Source: CAD feature listing. Evaluate the final solid. Frame: model axes, mm. Face numbers are marked on the shaded views. Give positions to 0.01 mm unless a question says otherwise; leave off trailing zeros. Loops run counter-clockwise (first coordinate to the right, second up) from the corner with the lowest first, then second, coordinate; pieces in that order, holes last.
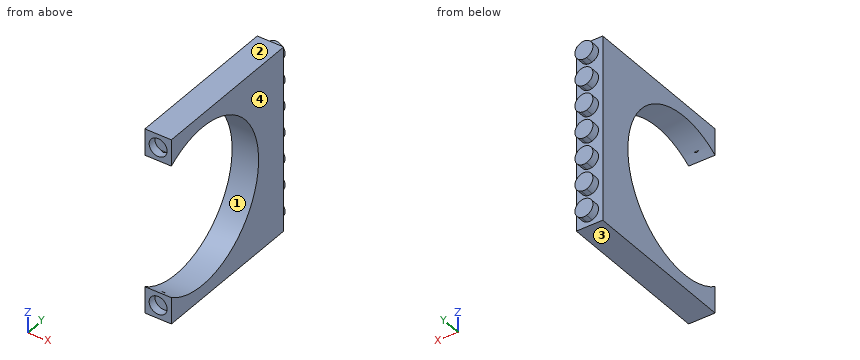
Autodesk Inventor part; units mm, degrees
ref_plane "YZ Plane" through (0, 0, 0) normal (1, 0, 0) x (0, 1, 0)
ref_plane "XZ Plane" through (0, 0, 0) normal (0, 1, 0) x (-1, 0, 0)
ref_plane "XY Plane" through (0, 0, 0) normal (0, 0, 1) x (1, 0, 0)
sketch "草圖1" plane through (0, 0, 0) normal (0, 1, 0) x (-1, 0, 0)
  line L0 (5, 0) -> (0, 0)
  line L1 (0, 0) -> (0, -35)
  line L2 (0, -35) -> (5, -35)
  line L3 (5, -35) -> (5, 0)
  circle A0 centre (2.5, -2.5) radius 1.7
  circle A1 centre (2.5, -7.5) radius 1.7
  circle A2 centre (2.5, -12.5) radius 1.7
  circle A3 centre (2.5, -17.5) radius 1.7
  circle A4 centre (2.5, -22.5) radius 1.7
  circle A5 centre (2.5, -27.5) radius 1.7
  circle A6 centre (2.5, -32.5) radius 1.7
  line L4 (5, -5) -> (0, -5)
  line L5 (5, -30) -> (0, -30)
  dimension "d0" = 5
  dimension "d1" = 35
  dimension "d2" = 3.4
  dimension "d3" = 2.5
  dimension "d4" = 2.5
  dimension "d7" = 5
  dimension "d12" = 5
  dimension "d13" = 5
sketch "草圖2" plane through (0, 0, 0) normal (1, 0, 0) x (0, 1, 0)
  line L0 (0, 0) -> (0, -35)
  line L1 (0, 0) -> (30, 0)
  line L2 (30, 0) -> (30, -35)
  line L3 (30, -35) -> (0, -35)
  arc A0 (0, -30) -> (0, -5) centre (8.2916, -17.5) ccw
  point P0 (0, -5)
  dimension "d15" = 30
  dimension "d25" = 15
extrude "擠出1" add sketch "草圖2" against normal blind 5 contours L1 L2 L3 L0 A0
extrude "擠出2" cut sketch "草圖1" along normal blind 1.5 contours A0 | A6
sketch "草圖3" plane through (0, 30, 0) normal (0, 1, 0) x (1, 0, 0)
  arc A0 (-2.9974, 4.1256) -> (-2.0026, 4.1256) centre (-2.5, 2.5) ccw
  circle A1 centre (-2.5, 2.5) radius 1.7
  point P0 (0, 0)
  point P1 (-2.9974, 4.1256)
extrude "擠出4" add sketch "草圖3" along normal blind 1.5
pattern_linear "矩形陣列2" count 7 spacing 5 along (0, 0, -1) of "擠出4"
properties part number "110033226_ipt_22_塔樓門口"
(1) Section A-A, the plane y = 17. Return the cut outline in (x, z), then the cut area to 3 significant figures.
A:
outline: (-5, -35) - (0, -35) - (0, -29.71) - (-5, -29.71) - close; (-5, -5.29) - (0, -5.29) - (0, 0) - (-5, 0) - close
area: 52.9 mm2
(2) Section C-C, the plane x = -2.5. Count the separate pieces of the cut face and the enclosed holes in it, then the cut area to 3 significant figures.
A:
separate pieces: 3
enclosed holes: 0
area: 487 mm2
(3) Ray query, line 1 along Z through (x, y) = (-2.5, 0.45); line 2 along Z through (x, y) = (-2.5, 0.6); line 3 along X through (y, z) = (1.1, -2.5). Return the intervals inside material, ascending.
A:
line 1: z = -35 to -34.2, -30.8 to -30.29, -4.71 to -4.2, -0.8 to 0
line 2: z = -35 to -34.2, -30.8 to -30.38, -4.62 to -4.2, -0.8 to 0
line 3: x = -5 to -4.2, -0.8 to 0
(4) Mould query, pull axis Z, two halves, no side actions, for the marked faces 1, 2, 3 and 4. Classes: pulls with the +Z half, pulls with the -Z half, needs draft (parallel to the pull), parting line crosses it, or undercut.
A:
face 1: undercut
face 2: pulls with the +Z half
face 3: pulls with the -Z half
face 4: needs draft
(5) First-contact query: pin 1 (1 mm diameter, centred on x = -3, z = -33, fed in from -Y); pin 2 (1 mm diameter, centred on x = -2.5, z = -29, fed in from -Y). Flat tips, straight axial feed; report the tip coordinate or a pass-through.
A:
pin 1: stops at y = 1.5
pin 2: stops at y = 17.29
(6) Section D-D, the plane z = -27.5. Return the cut outline in (x, y), then the cut area to 3 significant figures.
A:
outline: (-5, 19.47) - (0, 19.47) - (0, 30) - (-0.8, 30) - (-0.8, 31.5) - (-4.2, 31.5) - (-4.2, 30) - (-5, 30) - close
area: 57.7 mm2
(7) Section B-B, the plane z = -23.5. Return the cut outline in (x, y), then the cut area to 3 significant figures.
A:
outline: (-5, 22.04) - (0, 22.04) - (0, 30) - (-1.13, 30) - (-1.13, 31.5) - (-3.87, 31.5) - (-3.87, 30) - (-5, 30) - close
area: 43.9 mm2
